Geometry: final body of the model. Coordinates: model frame, mm. A direction names the side the tool comes from. Coordinates: 2 decimals unless noted, no trailing zeros. Loops run counter-clockwise (first coordinate to the right, second up) from the corner with the lowest first, then second, coordinate; pieces in that order, holes last. Notation, with made-up numbers: (3.5, -13.5) - (29.5, -13.5) arc R22 cw to (29.5, 2.5) - close; hole circle Ø5 at (79.5, 86). An arc over 180 degrees is marked (long way). Return JSON: item names as keys, results as strings.
Autodesk Inventor part; units mm, degrees
ref_plane "YZ Plane" through (0, 0, 0) normal (1, 0, 0) x (0, 1, 0)
ref_plane "XZ Plane" through (0, 0, 0) normal (0, 1, 0) x (-1, 0, 0)
ref_plane "XY Plane" through (0, 0, 0) normal (0, 0, 1) x (1, 0, 0)
sketch "Sketch1" plane through (0, 0, 0) normal (0, 1, 0) x (-1, 0, 0)
  circle A0 centre (0, 0) radius 5.9055
  dimension "d0" = 11.811
extrude "Extrusion1" add sketch "Sketch1" along normal blind 0.508
sketch "Sketch2" plane through (0, 0.508, 0) normal (0, 1, 0) x (1, 0, 0)
  line L0 (-6.0608, 1.4528) -> (-1.7723, 5.9752)
  line L1 (-1.7723, 5.9752) -> (4.2885, 4.5224)
  line L2 (4.2885, 4.5224) -> (6.0608, -1.4528)
  line L3 (6.0608, -1.4528) -> (1.7723, -5.9752)
  line L4 (1.7723, -5.9752) -> (-4.2885, -4.5224)
  line L5 (-4.2885, -4.5224) -> (-6.0608, 1.4528)
  point P0 (0, 0)
  point P1 (0, 0)
  dimension "d3" = 10.795
extrude "Extrusion2" add sketch "Sketch2" along normal blind 1.524
sketch "Sketch3" plane through (0, 0, 0) normal (0, -1, 0) x (1, 0, 0)
  circle A0 centre (0, 0) radius 3.175
  dimension "d6" = 6.35
extrude "Extrusion3" add sketch "Sketch3" against normal blind 3.4544
sketch "Sketch4" plane through (0, 3.4544, 0) normal (0, 1, 0) x (1, 0, 0)
  circle A0 centre (0, 0) radius 2.9845
  dimension "d9" = 5.969
extrude "Extrusion4" add sketch "Sketch4" along normal blind 8.89
sketch "Sketch5" plane through (0, 12.3444, 0) normal (0, 1, 0) x (1, 0, 0)
  line L0 (-3.3844, -0.254) -> (-2.4365, 0)
  line L1 (-2.4365, 0) -> (-3.3844, 0.254)
  line L2 (-3.3844, 0.254) -> (-3.3844, -0.254)
  line L3 (0, 0) -> (-2.1237, 0)
  dimension "d12" = 30
  dimension "d13" = 0.508
  dimension "d14" = 0.254
extrude "Extrusion5" cut sketch "Sketch5" against normal blind 8.89
pattern_circular "Circular Pattern2" count 25 over 360 about axis through (0, 3.4544, 0) along (0, 1, 0) of "Extrusion5"
sketch "Sketch6" plane through (0, 12.3444, 0) normal (0, 1, 0) x (1, 0, 0)
  line L0 (0.5715, -4.3158) -> (-0.5715, -4.3158)
  line L1 (-0.5715, -4.3158) -> (-0.5715, 4.3783)
  line L2 (-0.5715, 4.3783) -> (0.5715, 4.3783)
  line L3 (0.5715, 4.3783) -> (0.5715, -4.3158)
  point P0 (0, 0)
  dimension "d23" = 1.143
  dimension "d24" = 0.5715
extrude "Extrusion6" cut sketch "Sketch6" against normal blind 8.89
equation "\"d14\" = 0.5 * d13"
properties part number "Button_Knob" material "Stainless Steel"
Item 1: First-contact query: pin 1 Ø2 at (y, z) = (8, 2) entering from +X; pin 2 Ø2 at (x, z) = (2, -3.5) entering from +Y; pin 3 Ø2.5 at (x, z) = (4, 4) entering from +Y. Flat tips, straight axial feed; report the tip coordinate or a pass-through.
Worked out:
{"pin 1": "x = 2.72", "pin 2": "y = 3.45", "pin 3": "y = 2.03"}
Item 2: Reachability of faces 1 (the face through (-1.25, 0.508, 5.44)), 2 (the face through (1.3, 0.508, -5.4)), 3 (the face through (4, 0.508, 4)), 4 (the face through (-3.95, 1.26, -3.68)) from +Z, -Z, +X, -X, +Y, -Y: full face, straight path, thin tool, end or side. Return the list, or none.
Worked out:
{"face 1": "+Z, -X, +Y", "face 2": "-Z, +X, +Y", "face 3": "+Z, +X, +Y", "face 4": "-Z, -X, +Y"}
Item 3: Section query B-B, the plane z = 3.5. Return loops of the section in (x, y).
Worked out:
{"outline": "(-4.76, 0) - (4.76, 0) - (4.76, 0.51) - (4.12, 0.51) - (4.12, 2.03) - (-4.59, 2.03) - (-4.59, 0.51) - (-4.76, 0.51) - close"}
Item 4: Ray query, probe 1 along Y at (x, z) = (0, -3.5); probe 2 along X at (y, z) = (10.75, 1); probe 3 along X at (y, z) = (2.25, -2). Return the intervals inside material, ascending. Write a range as from..to.
Worked out:
{"probe 1": "0..2.03", "probe 2": "-2.81..-0.57, 0.57..2.4", "probe 3": "-2.47..2.47"}
Item 5: Section query A-A, the plane x = 5. Return loops of the section in (y, z), and give its area (3 significant figures).
Worked out:
{"outline": "(0, -3.14) - (0.51, -3.14) - (0.51, -2.12) - (2.03, -2.12) - (2.03, 2.57) - (0.51, 2.57) - (0.51, 3.14) - (0, 3.14) - close", "area": "10.3 mm^2"}
Item 6: Mould query, pull axis X, two halves, no side actions, for faces 5 (the face through (-0.69, 2.73, -3.1)), 6 (the face through (-0.572, 8, 0)), 7 (the face through (0.572, 8, 0)), 8 (the face through (1, 12.344, 0)). Classes: +X half, -X half, draft (parallel to the pull), parting line (faces both ways), or undercut.
Worked out:
{"face 5": "parting line", "face 6": "undercut", "face 7": "undercut", "face 8": "draft"}
